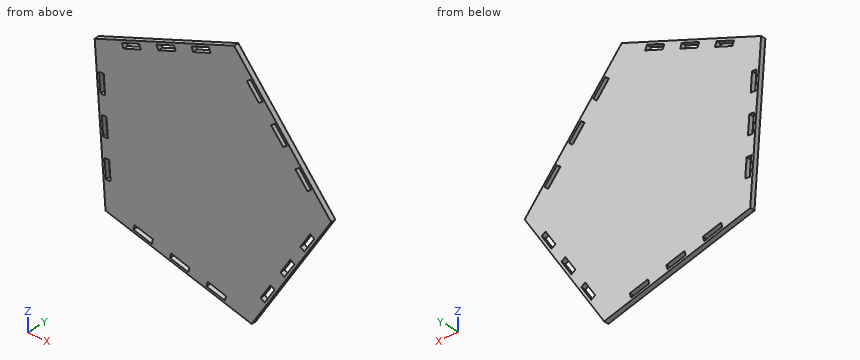
```python
from build123d import *

# Parameters (mm, degrees)
BOSS_EXTRUDE1_DEPTH = 6.35
CUT_EXTRUDE1_DEPTH  = 7.35
CUT_EXTRUDE2_DEPTH  = 7.35
CUT_EXTRUDE3_DEPTH  = 7.35
CUT_EXTRUDE4_DEPTH  = 7.35
CUT_EXTRUDE5_DEPTH  = 7.35


with BuildPart() as part:
    # Sketch1 → Boss-Extrude1 (new body)
    with BuildSketch(Plane(origin=(0, 0, 0), x_dir=(1, 0, 0), z_dir=(0, 1, 0))):
        Polygon((-472.762098838, -38.601599313), (-579.996957803, 133.998878735), (-777.287160977, 85.348948297), (-791.984353221, -117.318840313), (-603.777514393, -193.924491661), align=None)
    extrude(amount=BOSS_EXTRUDE1_DEPTH)

    # Sketch2 → Cut-Extrude1 (cut, through all)
    with BuildSketch(Plane(origin=(0, 6.35, 0), x_dir=(1, 0, 0), z_dir=(0, 1, 0))):
        Polygon((-659.001261619, -161.163030045), (-635.475406766, -170.738736463), (-637.86933337, -176.620200176), (-661.395188224, -167.044493758), align=None)
        Polygon((-706.052971326, -142.011617208), (-682.527116473, -151.587323626), (-684.921043077, -157.46878734), (-708.446897931, -147.893080921), align=None)
        Polygon((-753.053854552, -122.735332494), (-729.527999698, -132.311038913), (-731.921926303, -138.192502626), (-755.447781156, -128.616796208), align=None)
    extrude(amount=-CUT_EXTRUDE1_DEPTH, mode=Mode.SUBTRACT)

    # Sketch4 → Cut-Extrude2 (cut, through all)
    with BuildSketch(Plane(origin=(0, 6.35, 0), x_dir=(1, 0, 0), z_dir=(0, 1, 0))):
        Polygon((-570.115957611, -139.244740198), (-565.262117225, -143.338971934), (-581.639044169, -162.754333478), (-586.492884555, -158.660101741), align=None)
        Polygon((-520.985176778, -80.998655568), (-516.131336392, -85.092887304), (-499.754409447, -65.677525761), (-504.608249833, -61.583294024), align=None)
        Polygon((-548.88519028, -123.923610391), (-532.508263336, -104.508248847), (-537.362103722, -100.414017111), (-553.739030666, -119.829378655), align=None)
    extrude(amount=-CUT_EXTRUDE2_DEPTH, mode=Mode.SUBTRACT)

    # Sketch5 → Cut-Extrude3 (cut, through all)
    with BuildSketch(Plane(origin=(0, 6.35, 0), x_dir=(1, 0, 0), z_dir=(0, 1, 0))):
        Polygon((-777.891428053, -54.674087259), (-784.224796447, -54.214800001), (-786.061945478, -79.548273578), (-779.728577084, -80.007560835), align=None)
        Polygon((-774.217129992, -4.007140106), (-780.550498387, -3.547852849), (-782.387647417, -28.881326425), (-776.054279023, -29.340613683), align=None)
        Polygon((-776.876200326, 47.119094304), (-770.542831932, 46.659807046), (-772.379980962, 21.32633347), (-778.713349356, 21.785620727), align=None)
    extrude(amount=-CUT_EXTRUDE3_DEPTH, mode=Mode.SUBTRACT)

    # Sketch6 → Cut-Extrude4 (cut, through all)
    with BuildSketch(Plane(origin=(0, 6.35, 0), x_dir=(1, 0, 0), z_dir=(0, 1, 0))):
        Polygon((-508.969874734, 13.660505405), (-495.565517364, -7.914554351), (-500.959282303, -11.265643693), (-514.363639673, 10.309416063), align=None)
        Polygon((-522.374232105, 35.235565162), (-527.767997044, 31.884475819), (-541.172354415, 53.459535575), (-535.778589476, 56.810624918), align=None)
        Polygon((-549.139796727, 78.412493389), (-554.533561666, 75.061404046), (-567.937919036, 96.636463802), (-562.544154097, 99.987553145), align=None)
    extrude(amount=-CUT_EXTRUDE4_DEPTH, mode=Mode.SUBTRACT)

    # Sketch7 → Cut-Extrude5 (cut, through all)
    with BuildSketch(Plane(origin=(0, 6.35, 0), x_dir=(1, 0, 0), z_dir=(0, 1, 0))):
        Polygon((-614.708405409, 115.629038504), (-639.369680806, 109.5477972), (-640.889991132, 115.713116049), (-616.228715735, 121.794357354), align=None)
        Polygon((-665.551266529, 109.631874744), (-690.212541925, 103.550633439), (-688.692231599, 97.38531459), (-664.030956203, 103.466555895), align=None)
        Polygon((-714.873817322, 97.469392134), (-739.535092719, 91.38815083), (-738.014782393, 85.22283198), (-713.353506996, 91.304073285), align=None)
    extrude(amount=-CUT_EXTRUDE5_DEPTH, mode=Mode.SUBTRACT)


solid = part.part
```
Verification items for the finished model (mm, model axes). Coordinates: 2 decimals unless noted, no trailing zeros. Write each loop counter-clockwise with the first axis right and the second up, starting at its lowest first coordinate (ties: lowest second). Pieces come first, ordered by that corner, then holes. Notation, with made-up numbers: M 7,1 L 59,1 A18 ccw 59,16 Z; hole C -9.5,22 d2. An arc over 180 degrees is marked long. Answer as a JSON object with one key per item and string values. Group by question number.
(1) Gauge pin test, flat ends, axial feed: pin 1 (1.5 mm diameter, centred on x = -515.5, y = 5.5, fed in from +Z); pin 2 (3 mm diameter, centred on x = -551.5, y = 5.5, fed in from -Z); pin 3 (1.5 mm diameter, centred on x = -652, y = 1, fed in from +Z). Record the tip position at first contact, or that the pin passes through.
(2) Cross-section at D-D, the plane x = -595.5. Record the cut outline in (y, z), and give its area (3 significant figures).
(3) Cross-section at A-A, the plane x = -545. Record the cut outline in (y, z).
(4) Cross-section at C-C, the plane x = -766.5. Record the cut outline in (y, z), and give its area (3 significant figures).
(5) Cross-section at B-B, the plane y = 3. State how many separate pieces and enclosed holes the cut face has, and give its area (3 significant figures).
(6) Material ranges on line 1 (Z direction, x = -505, y = 3); line 2 (X direction, y = 4.5, z = 133.5); line 3 (Z direction, x = -656.5, y = 1), recorded low to high.
Reply:
{
 "1": {"pin 1": "z = 90.16", "pin 2": "z = -90.55", "pin 3": "z = 174.6"},
 "2": {"outline": "M 0,-130.18 L 6.35,-130.18 L 6.35,184.11 L 0,184.11 Z", "area": "2,000 mm²"},
 "3": {"outline": "M 0,-77.67 L 6.35,-77.67 L 6.35,109.47 L 0,109.47 Z; M 0,119.32 L 6.35,119.32 L 6.35,124.24 L 0,124.24 Z"},
 "4": {"outline": "M 0,-88.01 L 6.35,-88.01 L 6.35,127.69 L 0,127.69 Z", "area": "1,370 mm²"},
 "5": {"separate pieces": "1", "enclosed holes": "15", "area": "68,600 mm²"},
 "6": {"line 1": "-13.29 to -7.27, 4.76 to 62.05, 71.9 to 76.82", "line 2": "-752.23 to -743.45, -730.01 to -552.81", "line 3": "-115.13 to 162.18, 169.04 to 172.46"}
}
